Verification items for the finished model (mm, model axes). A direction names the side the tool comes from. Coordinates: 2 decimals unless noted, no trailing zeros. Order: outer loops, then holes, each group sorted by start corner. A loop starts at its lowest first (then second) coordinate and runs counter-clockwise, first axis right, second up. Notation, with made-up numbers: (37, -8) - (41, -8) arc R25 ccw to (41, 7) - close; hole circle Ø8 at (86.5, 66.5). An arc over 180 degrees is marked (long way). One line per question, with ' | ' between items. Start each with the question number.
from build123d import *
from OCP.BRepFilletAPI import BRepFilletAPI_MakeChamfer

# Parameters (mm, degrees)
BOSS_EXTRUDE1_DEPTH     = 24
SKETCH2_R               = 2.5
CUT_EXTRUDE1_DEPTH      = 46.458222579
SKETCH3_W               = 62.6
SKETCH3_H               = 22.6
BOSS_EXTRUDE2_DEPTH     = 5
SKETCH4_W               = 30
SKETCH4_H               = 30
SKETCH4_W_2             = 20
SKETCH4_H_2             = 20
BOSS_EXTRUDE3_DEPTH     = 20
SKETCH6_W               = 20
SKETCH6_H               = 20
BOSS_EXTRUDE4_DEPTH     = 20
SKETCH8_W               = 2
SKETCH8_H               = 4.711017494
SKETCH8_W_2             = 4.711017494
SKETCH8_H_2             = 2
BOSS_EXTRUDE5_DEPTH     = 20
SKETCH9_W               = 5
SKETCH9_H               = 3.7
BOSS_EXTRUDE6_DEPTH     = 29
CHAMFER1_SIZE           = 29
CHAMFER1_SIZE2          = 3.7
CHAMFER3_SIZE           = 3.7
CHAMFER3_SIZE_2         = 5
CHAMFER4_SIZE           = 5
CHAMFER4_SIZE_2         = 3.7
CHAMFER5_SIZE2          = 3.7
CHAMFER5_SIZE           = 5
CUT_EXTRUDE2_DEPTH      = 45.33610267
CUT_EXTRUDE2_DEPTH_BACK = 45.33610267
SKETCH11_R              = 1.95


# Some blends are built 0.0001 mm under size
with BuildPart() as part:
    # Sketch1 → Boss-Extrude1 (new body)
    with BuildSketch(Plane(origin=(0, 0, 0), x_dir=(1, 0, 0), z_dir=(0, 1, 0))):
        Polygon((-13.7, -6.3), (-8.7, -11.3), (-31.3, -11.3), (-31.3, 11.3), (-8.7, 11.3), (-13.7, 6.3), (-26.3, 6.3), (-26.3, -6.3), align=None)
        Polygon((8.7, 11.3), (8.7, 0), (13.7, 0), (13.7, 6.3), (26.3, 6.3), (31.3, 11.3), align=None)
        Polygon((13.7, 0), (8.7, 0), (8.7, -11.3), (31.3, -11.3), (26.3, -6.3), (13.7, -6.3), align=None)
    extrude(amount=BOSS_EXTRUDE1_DEPTH)

    # Sketch2 → Cut-Extrude1 (cut, through all)
    with BuildSketch(Plane.XY.offset(11.3)):
        with Locations((-20, 19)):
            Circle(SKETCH2_R)
        with Locations((-20, 4.5)):
            Circle(SKETCH2_R)
        with Locations((20, 4.5)):
            Circle(SKETCH2_R)
        with Locations((20, 19)):
            Circle(SKETCH2_R)
    extrude(amount=-CUT_EXTRUDE1_DEPTH, mode=Mode.SUBTRACT)

    # Sketch3 → Boss-Extrude2 (add)
    with BuildSketch(Plane.XZ):
        Rectangle(SKETCH3_W, SKETCH3_H)
    extrude(amount=BOSS_EXTRUDE2_DEPTH)

    # Sketch4 → Boss-Extrude3 (add)
    with BuildSketch(Plane.XZ.offset(5)):
        Rectangle(SKETCH4_W, SKETCH4_H)
        Rectangle(SKETCH4_W_2, SKETCH4_H_2, mode=Mode.SUBTRACT)
    extrude(amount=BOSS_EXTRUDE3_DEPTH)

    # Sketch6 → Boss-Extrude4 (add)
    with BuildSketch(Plane.XZ.offset(25)):
        Polygon((15, 15), (31.3, 11.3), (31.3, -11.3), (15, -15), (-15, -15), (-31.3, -11.3), (-31.3, 11.3), (-15, 15), align=None)
        Rectangle(SKETCH6_W, SKETCH6_H, mode=Mode.SUBTRACT)
    extrude(amount=-BOSS_EXTRUDE4_DEPTH)

    # Sketch8 → Boss-Extrude5 (add)
    with BuildSketch(Plane.XZ.offset(5)):
        Polygon((4, 2.5), (4, -2.5), (8, -5), (8, -2.355508747), (8, 2.355508747), (8, 5), align=None)
        with Locations((9, 0)):
            Rectangle(SKETCH8_W, SKETCH8_H)
        with Locations((0, 9)):
            Rectangle(SKETCH8_W_2, SKETCH8_H_2)
        Polygon((5, 8), (2.355508747, 8), (-2.355508747, 8), (-5, 8), (-2.5, 4), (2.5, 4), align=None)
        with Locations((-9, 0)):
            Rectangle(SKETCH8_W, SKETCH8_H)
        Polygon((-8, 2.355508747), (-8, -2.355508747), (-8, -5), (-4, -2.5), (-4, 2.5), (-8, 5), align=None)
        with Locations((0, -9)):
            Rectangle(SKETCH8_W_2, SKETCH8_H_2)
        Polygon((-2.355508747, -8), (2.355508747, -8), (5, -8), (2.5, -4), (-2.5, -4), (-5, -8), align=None)
    extrude(amount=BOSS_EXTRUDE5_DEPTH)

    # Sketch9 → Boss-Extrude6 (add)
    with BuildSketch(Plane(origin=(0, -5, 0), x_dir=(1, 0, 0), z_dir=(0, 1, 0))):
        with Locations((11.2, 13.15)):
            Rectangle(SKETCH9_W, SKETCH9_H)
        with Locations((11.2, -13.15)):
            Rectangle(SKETCH9_W, SKETCH9_H)
        with Locations((-11.2, 13.15)):
            Rectangle(SKETCH9_W, SKETCH9_H)
        with Locations((-11.2, -13.15)):
            Rectangle(SKETCH9_W, SKETCH9_H)
    extrude(amount=BOSS_EXTRUDE6_DEPTH)

    # Chamfer1: one chamfer whose edges measure the first distance from different faces: ONE call of the kernel's chamfer builder (chamfer() names one face for all edges)
    chamfer1_edges_1 = [part.edges().sort_by_distance(p)[0] for p in [
        (11.2, 24, -15),
        (-11.2, 24, -15),
    ]]
    chamfer1_side_1 = [part.faces().sort_by_distance(p)[0] for p in [
        (0, -7.016853933, -15),
    ]]
    chamfer1_edges_2 = [part.edges().sort_by_distance(p)[0] for p in [
        (-11.2, 24, 15),
        (11.2, 24, 15),
    ]]
    chamfer1_side_2 = [part.faces().sort_by_distance(p)[0] for p in [
        (0, -7.016853933, 15),
    ]]
    chamfer1 = BRepFilletAPI_MakeChamfer(part.part.solid().wrapped)
    for e in chamfer1_edges_1:
        chamfer1.Add(CHAMFER1_SIZE, CHAMFER1_SIZE2, e.wrapped, chamfer1_side_1[0].wrapped)  # the first distance lies on this face
    for e in chamfer1_edges_2:
        chamfer1.Add(CHAMFER1_SIZE, CHAMFER1_SIZE2, e.wrapped, chamfer1_side_2[0].wrapped)  # the first distance lies on this face
    add(Compound.cast(chamfer1.Shape()), mode=Mode.REPLACE)

    # Chamfer3
    # the kernel refuses this chamfer: 5, 3.7 mm, written as the material it adds along each edge
    with BuildSketch(Plane(origin=(21.605348649, -5, -11.3), x_dir=(0, -0.04206007695140814, -0.9991150834247482), z_dir=(-1, 0, 0))) as chamfer3_piece_1_section:
        Polygon((CHAMFER3_SIZE * 0.999115083425, -CHAMFER3_SIZE * 0.0420600769514), (-CHAMFER3_SIZE_2 * 0.0420600769514, -CHAMFER3_SIZE_2 * 0.999115083425), (0, 0), align=None)
    chamfer3_piece_1 = extrude(amount=43.210697297, mode=Mode.PRIVATE)
    chamfer3_piece_1 = split(chamfer3_piece_1, bisect_by=Plane(origin=(13.7, -3.301546392, -12.48628866), z_dir=(-1, 0, 0)), keep=Keep.TOP, mode=Mode.PRIVATE)
    chamfer3_piece_1 = split(chamfer3_piece_1, bisect_by=Plane(origin=(-13.7, -3.301546392, -12.48628866), z_dir=(1, 0, 0)), keep=Keep.TOP, mode=Mode.PRIVATE)
    add(chamfer3_piece_1)

    # Chamfer4
    chamfer4_edges_1 = [part.edges().sort_by_distance(p)[0] for p in [
        (22.5, -5, 11.3),
    ]]
    chamfer4_side_1 = [part.faces().sort_by_distance(p)[0] for p in [
        (22.5, -4.926, 11.3),
    ]]
    chamfer4_edges_2 = [part.edges().sort_by_distance(p)[0] for p in [
        (-22.5, -5, 11.3),
    ]]
    chamfer4_side_2 = [part.faces().sort_by_distance(p)[0] for p in [
        (-22.5, -4.926, 11.3),
    ]]
    chamfer4_edges_3 = [part.edges().sort_by_distance(p)[0] for p in [
        (22.5, -5, -11.3),
    ]]
    chamfer4_side_3 = [part.faces().sort_by_distance(p)[0] for p in [
        (22.5, -5, -11.374),
    ]]
    chamfer4_edges_4 = [part.edges().sort_by_distance(p)[0] for p in [
        (-22.5, -5, -11.3),
    ]]
    chamfer4_side_4 = [part.faces().sort_by_distance(p)[0] for p in [
        (-22.5, -5, -11.374),
    ]]
    chamfer4 = BRepFilletAPI_MakeChamfer(part.part.solid().wrapped)
    for e in chamfer4_edges_1:
        chamfer4.Add(CHAMFER4_SIZE - 0.0001, CHAMFER4_SIZE_2 - 0.0001, e.wrapped, chamfer4_side_1[0].wrapped)
    for e in chamfer4_edges_2:
        chamfer4.Add(CHAMFER4_SIZE - 0.0001, CHAMFER4_SIZE_2 - 0.0001, e.wrapped, chamfer4_side_2[0].wrapped)
    for e in chamfer4_edges_3:
        chamfer4.Add(CHAMFER4_SIZE_2 - 0.0001, CHAMFER4_SIZE - 0.0001, e.wrapped, chamfer4_side_3[0].wrapped)
    for e in chamfer4_edges_4:
        chamfer4.Add(CHAMFER4_SIZE_2 - 0.0001, CHAMFER4_SIZE - 0.0001, e.wrapped, chamfer4_side_4[0].wrapped)
    add(Compound.cast(chamfer4.Shape()), mode=Mode.REPLACE)  # a hair under: the kernel refuses the full size

    # Chamfer5
    chamfer5_edges = [part.edges().sort_by_distance(p)[0] for p in [
        (0, -5, 11.3),
    ]]
    chamfer5_side = [part.faces().sort_by_distance(p)[0] for p in [
        (0, -4.926, 11.3),
    ]]
    chamfer(chamfer5_edges, length=CHAMFER5_SIZE - 0.0001, length2=CHAMFER5_SIZE2 - 0.0001, reference=chamfer5_side[0])  # a hair under: the kernel refuses the full size

    # Sketch11 → Cut-Extrude2 (cut, two sides: drawn at the far end of the back side and taken through both)
    with BuildSketch(Plane.XY.offset(-4).offset(-CUT_EXTRUDE2_DEPTH_BACK)):
        with Locations((0, -15)):
            Circle(SKETCH11_R)
    extrude(amount=CUT_EXTRUDE2_DEPTH + CUT_EXTRUDE2_DEPTH_BACK, mode=Mode.SUBTRACT)


solid = part.part
Item 1: Section check A-A (x = 0). Give the number of separate pieces and of enclosed holes in the cut face, then the cut area to 3 significant figures.
Item 2: Section check C-C (x = 21). Record the cut outline in (y, z).
Item 3: Thickness scan on probe 1 along Y at (x, z) = (-20, 9); probe 2 along X at (y, z) = (-19.5, -8.5); probe 3 along Z at (x, y) = (9, -11). Record the ranges inside material, lowest first. Write a range as from..to.
Item 4: Mould release check, pull along Z, two halves, no side actions. Record for faces 6 (the cylindrical face through (18.16, 20.69, 8.84)), 7 (the flat face through (-6, -15, 10)), 8 (the flat face through (11.165, 9.703, -13.124)): +Z half, -Z half, draft (parallel to the pull), parting line (faces both ways), or undercut.
Item 5: Section check B-B (y = 12). Record the cut outline in (x, z), then the cut area to 3 significant figures.
Item 6: Set-up check for faces 1 (the flat face through (-3.77, -14.86, 6.03)), 2 (the flat face through (0.122, -2.535, -13.176)), 3 (the cylindrical face through (-21.84, 20.69, 8.84)), 4 (the flat face through (-11, 12, 9)), 5 (the flat face through (-23.036, -12.675, -13.176)): record each of +Z, -Z, +X, -X, +Y, -Y from which the full face is reachable in a straight line by a thin tool's end or side.
Item 7: Section check D-D (y = -3). Record the cut outline in (x, z), then the cut area to 3 significant figures.
Item 8: Gauge pin test, flat ends, axial feed: pin 1 (14 mm diameter, centred on x = 17.5, y = 9.5, fed in from +Z); pin 2 (4 mm diameter, centred on x = 20, y = 19, fed in from -Z); pin 3 (6 mm diameter, centred on x = -23.5, y = 15.5, fed in from -Z); pin 4 (3 mm diameter, centred on x = -18, y = -17, fed in from -Z). Record the tip position at first contact, or that the pin passes through.
Completed:
1) separate pieces: 3 | enclosed holes: 0 | area: 486 mm^2
2) outline: (-25, -13.64) - (-3.16, -13.64) - (0, -11.3) - (2.21, -11.3) - (2.21, -6.3) - (0, -6.3) - (0, 6.3) - (2.21, 6.3) - (2.21, 11.3) - (0, 11.3) - (-3.16, 13.64) - (-25, 13.64) - close; (6.79, -11.3) - (16.71, -11.3) - (16.71, -6.3) - (6.79, -6.3) - close; (6.79, 6.3) - (16.71, 6.3) - (16.71, 11.3) - (6.79, 11.3) - close; (21.29, -11.3) - (24, -11.3) - (24, -6.3) - (21.29, -6.3) - close; (21.29, 6.3) - (24, 6.3) - (24, 11.3) - (21.29, 11.3) - close
3) probe 1: y = -25..2, 7..16.5, 21.5..24 | probe 2: x = -31.3..-10, -2.36..2.36, 10..31.3 | probe 3: z = -15..-10, -2.36..2.36, 10..15
4) face 6: draft | face 7: undercut | face 8: -Z half
5) outline: (-31.3, -11.3) - (-13.7, -11.3) - (-13.7, -12.83) - (-8.7, -12.83) - (-8.7, -11.3) - (-13.7, -6.3) - (-26.3, -6.3) - (-26.3, 6.3) - (-13.7, 6.3) - (-8.7, 11.3) - (-8.7, 12.83) - (-13.7, 12.83) - (-13.7, 11.3) - (-31.3, 11.3) - close; (8.7, -12.83) - (13.7, -12.83) - (13.7, -11.3) - (31.3, -11.3) - (26.3, -6.3) - (13.7, -6.3) - (13.7, 6.3) - (26.3, 6.3) - (31.3, 11.3) - (13.7, 11.3) - (13.7, 12.83) - (8.7, 12.83) - close | area: 559 mm^2
6) face 1: -Y | face 2: -Z, +Y | face 3: +Z, -Z | face 4: +Y | face 5: -Z, -X, +Y, -Y
7) outline: (-31.3, -11.3) - (-21.52, -13.52) - (-13.7, -13.52) - (-13.7, -14.74) - (-8.7, -14.74) - (-8.7, -13.52) - (8.7, -13.52) - (8.7, -14.74) - (13.7, -14.74) - (13.7, -13.52) - (21.52, -13.52) - (31.3, -11.3) - (31.3, 11.3) - (21.52, 13.52) - (13.7, 13.52) - (13.7, 14.74) - (8.7, 14.74) - (8.7, 13.52) - (-8.7, 13.52) - (-8.7, 14.74) - (-13.7, 14.74) - (-13.7, 13.52) - (-21.52, 13.52) - (-31.3, 11.3) - close | area: 1,670 mm^2
8) pin 1: stops at z = 13.9 | pin 2: passes through | pin 3: stops at z = -11.3 | pin 4: stops at z = -14.66
